Part model, mm, in its own coordinate system. Face numbers are marked on the shaded views. A direction names the side the tool comes from. Give positions to 0.01 mm unless a question says otherwise; leave off trailing zeros. Order: outer loops, then holes, each group sorted by start corner. A loop starts at its lowest first (then second) coordinate and runs counter-clockwise, first axis right, second up. Notation, with made-up numbers: (34, -32.75) - (68, -32.75) arc R10 cw to (68, -28.75) - close; hole circle Ø4 at (53.25, 58). An arc over 180 degrees is marked (long way). One line per item, written item: value.
```python
from build123d import *

# Parameters (mm, degrees)
SKETCH1_W             = 45.4
SKETCH1_H             = 27
BOSS_EXTRUDE1_DEPTH   = 6
SKETCH4_W             = 45.4
SKETCH4_H             = 6
BOSS_EXTRUDE2_DEPTH   = 50
FILLET3_R             = 10
F_3_0MM_DOWEL_HOLE1_D = 3
F_3_0MM_DOWEL_HOLE2_D = 3.2
F_3_0MM_DOWEL_HOLE3_D = 3.2


with BuildPart() as part:
    # Sketch1 → Boss-Extrude1 (new body)
    with BuildSketch(Plane(origin=(0, 0, 0), x_dir=(1, 0, 0), z_dir=(0, 1, 0))):
        with Locations((22.7, 13.5)):
            Rectangle(SKETCH1_W, SKETCH1_H)
    extrude(amount=BOSS_EXTRUDE1_DEPTH)

    # Sketch4 → Boss-Extrude2 (add)
    with BuildSketch(Plane(origin=(0, 6, 0), x_dir=(1, 0, 0), z_dir=(0, 1, 0))):
        with Locations((22.7, 13.5)):
            Rectangle(SKETCH4_W, SKETCH4_H)
    extrude(amount=BOSS_EXTRUDE2_DEPTH)

    # Fillet3
    fillet3_edges = [part.edges().sort_by_distance(p)[0] for p in [
        (22.7, 6, -10.5),
        (22.7, 6, -16.5),
    ]]
    fillet(fillet3_edges, radius=FILLET3_R)

    # Ø3.0mm Dowel Hole1 (through all)
    with Locations(Plane(origin=(0, 16, 0), x_dir=(1, 0, 0), z_dir=(0, 1, 0))):
        with Locations((12.7, 23.5), (32.7, 23.5), (32.7, 3.5), (12.7, 3.5)):
            Hole(F_3_0MM_DOWEL_HOLE1_D / 2)

    # Ø3.0mm Dowel Hole2 (through all)
    with Locations(Plane(origin=(0, 0, -16.5), x_dir=(-1, 0, 0), z_dir=(0, 0, -1))):
        with Locations((-29.85, 50), (-15.55, 50)):
            Hole(F_3_0MM_DOWEL_HOLE2_D / 2)

    # Ø3.0mm Dowel Hole3 (through all)
    with Locations(Plane(origin=(4.2, 44, -16.5), x_dir=(-1, 0, 0), z_dir=(0, 0, -1))):
        with Locations((0, 0), (-37, 0)):
            Hole(F_3_0MM_DOWEL_HOLE3_D / 2)


solid = part.part
```
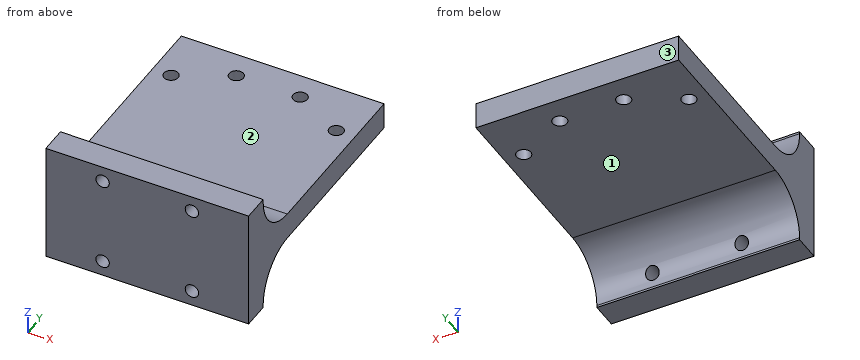
1) Slice it at A-A on x = 41.2. Write the cut outline in (y, z).
Answer:
outline: (0, -27) - (6, -27) - (6, -26.5) arc R10 cw to (16, -16.5) - (42.4, -16.5) - (42.4, -10.5) - (16, -10.5) arc R10 cw to (6, -0.5) - (6, 0) - (0, 0) - close; (45.6, -16.5) - (56, -16.5) - (56, -10.5) - (45.6, -10.5) - close
2) Drop flat-ended pins along their axis: P1, Ø10, axis at x = 12.5, y = 31, coming from the -Z side; P2, Ø4, axis at x = 4.2, y = 44, coming from the +Z side; P3, Ø5, axis at x = 12.7, z = -3.5, coming from the +Y side. Give the stop position or say it passes through.
Answer:
P1: stops at z = -16.5
P2: stops at z = -10.5
P3: stops at y = 7.65
3) Slice it at C-C on y = 14.5. Write the cut outline in (x, z), then the cut area to 3 significant figures.
Answer:
outline: (0, -16.61) - (45.4, -16.61) - (45.4, -10.39) - (0, -10.39) - close
area: 283 mm2
4) Wall check: line 1 along Z through (x, y) = (32.7, 3.25); line 2 along X through (y, z) = (4.75, -23.5); line 3 along Y through (x, z) = (4.2, -11.95). Give the ranges that are in metal, low to high. Write a range as [from, to].
Answer:
line 1: z = [-27, -25], [-22, -5], [-2, 0]
line 2: x = [0, 11.2], [14.2, 31.2], [34.2, 45.4]
line 3: y = [0, 42.4], [45.6, 56]
5) Slice it at B-B on z = -2.75. Write the cut outline in (x, y), then the cut area to 3 significant figures.
Answer:
outline: (0, 0) - (11.4, 0) - (11.4, 6.26) - (0, 6.26) - close; (14, 0) - (31.4, 0) - (31.4, 6.26) - (14, 6.26) - close; (34, 0) - (45.4, 0) - (45.4, 6.26) - (34, 6.26) - close
area: 252 mm2
6) Slice it at D-D on z = -18.5. Write the cut outline in (x, y).
Answer:
outline: (0, 0) - (45.4, 0) - (45.4, 10) - (0, 10) - close
7) Which spindle directions (+Z, -Z, +X, -X, +Y, -Y) get a long thin tool onto all of the face, cutting with end or side? Do the marked faces 1, 2 and 3. Say none if no direction does.
Answer:
face 1: -Z, +X, -X, +Y
face 2: +Z, +X, -X, +Y
face 3: +Z, -Z, +X, -X, +Y
